Here's how the part is built. I have some questions about the finished solid (model axes, mm). A direction names the side the tool comes from. Round coordinates to 2 decimals unless told otherwise and drop trailing zeros. Write each loop counter-clockwise with the first axis right and the second up, starting at its lowest first coordinate (ties: lowest second). Pieces come first, ordered by that corner, then holes. Notation, with made-up numbers: M -19,45 L 20,45 A28 ccw 20,80 Z; hole C 16.25,0.25 d1. An arc over 180 degrees is marked long. Write item = value, one per line. Start each with the question number.
(1) I want a section at B-B (x = 0). List the corners of the cut face in (y, z) for me, and give its area (3 significant figures).
(2) I want a section at A-A (z = -20). List the corners of the cut face in (x, y) for me.
(3) I want a section at C-C (x = -16.6). List the corners of the cut face in (y, z) for me, and give its area (3 significant figures).
(4) Will these pins go through, and if not, where does the flat tip stop? pin 1 Ø1 at (y, z) = (2.5, 1) entering from +X; pin 2 Ø3 at (x, y) = (27.5, 2) entering from +Z; pin 3 Ø2 at (x, y) = (-6, 1) entering from +Z.
(5) If we mould it in two halves opening along Z, with no side actions, what happens to faces 1 (the cylindrical face through (-32.1, 2.54, -15.86)), 2 (the cylindrical face through (10.796, 2.465, 17.3)), 3 (the flat face through (23, 2, 2)), 4 (the cylindrical face through (-20.02, 2.54, 12.04))? For each: released by +Z, released by -Z, zero draft, split by the parting line, or undercut.
(6) On a 3-axis mill with a long thin cutter (end or side, diameter ignored), from which of +Z, -Z, +X, -X, +Y, -Y can I reach the whole of each face in a straight line? I mean faces 5 (the flat face through (0, 0, -16)), 6 (the flat face through (-23, 2, 2)), 7 (the cylindrical face through (-18.24, 2.46, 21.41)). Say none if no direction works.
(7) I want a section at D-D (y = 1.8). Give the number of separate pieces and of enclosed holes in the cut face, and give its area (3 significant figures).
(8) I need wall thicknesses on line 1 along X through (y, z) = (2.35, -20); line 2 along X through (y, z) = (0.6, 16); line 3 along Z through (x, y) = (-7.5, 2.15). Which ranges of each line are inside material? Lowest first, please.
```python
from build123d import *

# Parameters (mm, degrees)
SKETCH_1_W          = 46
SKETCH_1_H          = 70
EXTRUDE_1_DEPTH     = 5
SKETCH_2_R          = 4
CUT_EXTRUDE_1_DEPTH = 43.178193418
FILLET_1_R          = 20
CUT_EXTRUDE_4_DEPTH = 43.178193418
FILLET_3_R          = 3
SKETCH_8_W          = 20
SKETCH_8_H          = 5
EXTRUDE_2_DEPTH     = 10
SKETCH_9_W          = 20
SKETCH_9_H          = 5
EXTRUDE_3_DEPTH     = 10
FILLET_6_R          = 3
SKETCH_10_R         = 1.5
CUT_EXTRUDE_5_DEPTH = 49.363209157
SKETCH_11_W         = 30
SKETCH_11_H         = 10
CUT_EXTRUDE_6_DEPTH = 49.363209157
FILLET_7_R          = 3


with BuildPart() as part:
    # 草图1 → 凸台-拉伸1 (new body)
    with BuildSketch(Plane(origin=(0, 0, 0), x_dir=(1, 0, 0), z_dir=(0, 1, 0))):
        Rectangle(SKETCH_1_W, SKETCH_1_H)
    extrude(amount=EXTRUDE_1_DEPTH)

    # 草图2 → 切除-拉伸1 (cut, through all)
    with BuildSketch(Plane.XZ):
        with Locations(Location((0, 11, 0), (0, 0, 270))):
            Circle(SKETCH_2_R)
    extrude(amount=-CUT_EXTRUDE_1_DEPTH, mode=Mode.SUBTRACT)

    # 圆角1
    fillet_1_edges = [part.edges().sort_by_distance(p)[0] for p in [
        (23, 2.5, 35),
        (-23, 2.5, 35),
    ]]
    fillet(fillet_1_edges, radius=FILLET_1_R)

    # 草图6 → 切除-拉伸4 (cut, through all)
    with BuildSketch(Plane.XZ):
        with BuildLine():
            Line((12.5, 11), (21, 11))
            ThreePointArc((21, 11), (18.186533479, 21.5), (10.5, 29.186533479))
            Line((10.5, 29.186533479), (6.25, 21.825317547))
            ThreePointArc((6.25, 21.825317547), (10.825317547, 17.25), (12.5, 11))
        make_face()
        with BuildLine():
            Line((-12.5, 11), (-21, 11))
            ThreePointArc((-21, 11), (-18.186533479, 21.5), (-10.5, 29.186533479))
            Line((-10.5, 29.186533479), (-6.25, 21.825317547))
            ThreePointArc((-6.25, 21.825317547), (-10.825317547, 17.25), (-12.5, 11))
        make_face()
    extrude(amount=-CUT_EXTRUDE_4_DEPTH, mode=Mode.SUBTRACT)

    # 圆角3
    fillet_3_edges = [part.edges().sort_by_distance(p)[0] for p in [
        (-6.25, 2.5, 21.825317547),
        (-12.5, 2.5, 11),
        (-21, 2.5, 11),
        (-10.5, 2.5, 29.186533479),
        (12.5, 2.5, 11),
        (6.25, 2.5, 21.825317547),
        (10.5, 2.5, 29.186533479),
        (21, 2.5, 11),
    ]]
    fillet(fillet_3_edges, radius=FILLET_3_R)

    # 草图8 → 凸台-拉伸2 (add)
    with BuildSketch(Plane(origin=(23, 0, 0), x_dir=(0, 0, -1), z_dir=(1, 0, 0))):
        with Locations((25, 2.5)):
            Rectangle(SKETCH_8_W, SKETCH_8_H)
    extrude(amount=EXTRUDE_2_DEPTH)

    # 草图9 → 凸台-拉伸3 (add)
    with BuildSketch(Plane.ZY.offset(23)):
        with Locations((-25, 2.5)):
            Rectangle(SKETCH_9_W, SKETCH_9_H)
    extrude(amount=EXTRUDE_3_DEPTH)

    # 圆角6
    fillet_6_edges = [part.edges().sort_by_distance(p)[0] for p in [
        (23, 2.5, -15),
        (33, 2.5, -35),
        (33, 2.5, -15),
        (-23, 2.5, -15),
        (-33, 2.5, -35),
        (-33, 2.5, -15),
    ]]
    fillet(fillet_6_edges, radius=FILLET_6_R)

    # 草图10 → 切除-拉伸5 (cut, through all)
    with BuildSketch(Plane(origin=(0, 5, 0), x_dir=(1, 0, 0), z_dir=(0, 1, 0))):
        with Locations(Location((-16.6, 30, 0), (0, 0, 270))):
            Circle(SKETCH_10_R)
        with Locations(Location((0, 30, 0), (0, 0, 270))):
            Circle(SKETCH_10_R)
        with Locations(Location((16.6, 30, 0), (0, 0, 270))):
            Circle(SKETCH_10_R)
        with Locations(Location((16.6, 20, 0), (0, 0, 90))):
            Circle(SKETCH_10_R)
        with Locations(Location((0, 20, 0), (0, 0, 90))):
            Circle(SKETCH_10_R)
        with Locations(Location((-16.6, 20, 0), (0, 0, 90))):
            Circle(SKETCH_10_R)
    extrude(amount=-CUT_EXTRUDE_5_DEPTH, mode=Mode.SUBTRACT)

    # 草图11 → 切除-拉伸6 (cut, through all)
    with BuildSketch(Plane(origin=(0, 5, 0), x_dir=(1, 0, 0), z_dir=(0, 1, 0))):
        with Locations((0, 5)):
            Rectangle(SKETCH_11_W, SKETCH_11_H)
    extrude(amount=-CUT_EXTRUDE_6_DEPTH, mode=Mode.SUBTRACT)

    # 圆角7
    fillet_7_edges = [part.edges().sort_by_distance(p)[0] for p in [
        (15, 2.5, -10),
        (15, 2.5, 0),
        (-15, 2.5, 0),
        (-15, 2.5, -10),
    ]]
    fillet(fillet_7_edges, radius=FILLET_7_R)


solid = part.part
```
Returned:
q1.outline = M 0,-35 L 5,-35 L 5,-31.5 L 0,-31.5 Z; M 0,-28.5 L 5,-28.5 L 5,-21.5 L 0,-21.5 Z; M 0,-18.5 L 5,-18.5 L 5,-10 L 0,-10 Z; M 0,0 L 5,0 L 5,7 L 0,7 Z; M 0,15 L 5,15 L 5,35 L 0,35 Z
q1.area = 230 mm²
q2.outline = M -33,0 L -18.1,0 L -18.1,5 L -33,5 Z; M -15.1,0 L -1.5,0 L -1.5,5 L -15.1,5 Z; M 1.5,0 L 15.1,0 L 15.1,5 L 1.5,5 Z; M 18.1,0 L 33,0 L 33,5 L 18.1,5 Z
q3.outline = M 0,-35 L 5,-35 L 5,-31.5 L 0,-31.5 Z; M 0,-28.5 L 5,-28.5 L 5,-21.5 L 0,-21.5 Z; M 0,-18.5 L 5,-18.5 L 5,11 L 0,11 Z; M 0,23.86 L 5,23.86 L 5,29.66 L 0,29.66 Z
q3.area = 229 mm²
q4.pin_1 = 23
q4.pin_2 = -15
q4.pin_3 = 34.9
q5.face_1 = released by +Z
q5.face_2 = undercut
q5.face_3 = zero draft
q5.face_4 = undercut
q6.face_5 = +Z, -Z, +X, -X, -Y
q6.face_6 = +Z, -X, +Y, -Y
q6.face_7 = +Y, -Y
q7.separate_pieces = 1
q7.enclosed_holes = 10
q7.area = 2,780 mm²
q8.line_1 = -33 to -18.1, -15.1 to -1.5, 1.5 to 15.1, 18.1 to 33
q8.line_2 = -22.97 to -20.4, -11.46 to 11.46, 20.4 to 22.97
q8.line_3 = -35 to -10, 0 to 21.37, 23.97 to 34.49
